Part model, mm, in its own coordinate system. A direction names the side the tool comes from. Round coordinates to 2 decimals unless told otherwise and drop trailing zeros. Loops run counter-clockwise (first coordinate to the right, second up) from the corner with the lowest first, then second, coordinate; pieces in that order, holes last. Notation, with made-up numbers: M -25.75,80.25 L 29.25,80.25 A24 ccw 29.25,111.25 Z; hole C 30,-17.75 d10. An arc over 180 degrees is marked long. Write each question's results on one line, items separated by ' | '.
Autodesk Inventor part; units mm, degrees
ref_plane "YZ Plane" through (0, 0, 0) normal (1, 0, 0) x (0, 1, 0)
ref_plane "XZ Plane" through (0, 0, 0) normal (0, 1, 0) x (-1, 0, 0)
ref_plane "XY Plane" through (0, 0, 0) normal (0, 0, 1) x (1, 0, 0)
sketch "Base" plane through (0, 0, 0) normal (0, 0, 1) x (1, 0, 0)
  line L0 (0, 0) -> (-33.5334, -57.9479)
  line L1 (22.7363, 2.3748) -> (0, 0)
  line L2 (68.7163, -13.2577) -> (22.7363, 2.3748)
  line L3 (-33.5334, -57.9479) -> (-26.9158, -67.5067)
  line L4 (-26.9158, -67.5067) -> (-51.547, -128.5125)
  line L5 (-51.547, -128.5125) -> (-33.4114, -135.8348)
  line L6 (-26.9158, -67.5067) -> (12.6221, -101.6388) construction
  line L7 (12.6221, -101.6388) -> (22.7363, -101.0656)
  line L8 (12.6221, -101.6388) -> (-8.1441, -124.1457)
  line L9 (-33.4114, -135.8348) -> (-8.1441, -124.1457)
  line L10 (22.7363, 2.3748) -> (68.7163, -13.2577)
  line L11 (68.7163, -13.2577) -> (112.7039, -111.8391)
  line L12 (22.7363, 2.3748) -> (22.7363, -101.0656) construction
  line L13 (22.7363, -101.0656) -> (65.9464, -171.4033)
  line L14 (112.7039, -111.8391) -> (105.2475, -122.1197)
  line L15 (22.7363, -101.0656) -> (112.7039, -111.8391) construction
  line L16 (105.2475, -122.1197) -> (103.571, -134.8197)
  line L17 (103.571, -134.8197) -> (108.4402, -146.5492)
  line L18 (65.9464, -171.4033) -> (74.9694, -180.3406)
  line L19 (108.4402, -146.5492) -> (74.9694, -180.3406)
  circle A0 centre (85.3652, -157.1655) radius 25.4
  line L20 (-42.4792, -132.1736) -> (22.7363, -49.3454) construction
  line L21 (-33.0514, -120.1997) -> (-25.1949, -110.2215) construction
  line L22 (-35.546, -118.2356) -> (-27.6895, -108.2573)
  line L23 (-22.7004, -112.1856) -> (-30.5568, -122.1638)
  arc A1 (-35.546, -118.2356) -> (-30.5568, -122.1638) centre (-33.0514, -120.1997) ccw
  arc A2 (-22.7004, -112.1856) -> (-27.6895, -108.2573) centre (-25.1949, -110.2215) ccw
  circle A3 centre (85.3652, -157.1655) radius 4
  line L24 (0, -219.5535) -> (0, 39.3628)
  point P0 (-29.1232, -115.2106)
  point P1 (60.5618, -162.6381)
  dimension "d4" = 50.8
  dimension "d5" = 22.86
  dimension "d6" = 155.26
  dimension "d7" = 126.02
  dimension "d8" = 48.5647
  dimension "d9" = 66.9511
  dimension "d10" = 132.824
  dimension "d11" = 107.95
  dimension "d12" = 115.248
  dimension "d13" = 11.6259
  dimension "d14" = 65.7906
  dimension "d15" = 19.558
  dimension "d16" = 120
  dimension "d17" = 12.7
  dimension "d18" = 12.7
  dimension "d19" = 12.7
  dimension "d20" = 82.55
  dimension "d21" = 12.7
  dimension "d24" = 15.24
  dimension "d25" = 3.175
  dimension "d26" = 12.7
  dimension "d31" = 8
  dimension "d32" = 95.963
  dimension "d33" = 38.215
  dimension "d34" = 22.545
  dimension "d35" = 7.52
  dimension "d36" = 44.727
  dimension "d37" = 31.563
  dimension "d38" = 86.757
  dimension "d39" = 42.697
  dimension "d40" = 49.197
  dimension "d41" = 114.826
  dimension "d47" = 105.4209
  dimension "d48" = 62.051
extrude "Plate1" add sketch "Base" along normal blind 5
fillet "OutsideFilletsFeature" radius 6.35 14 edges at (68.7163, -13.2577, 2.5) (22.7363, 2.3748, 2.5) (0, 0, 2.5) (-33.5334, -57.9479, 2.5) (-26.9158, -67.5067, 2.5) (-51.547, -128.5125, 2.5) (-33.4114, -135.8348, 2.5) (-8.1441, -124.1457, 2.5) (12.6221, -101.6388, 2.5) (22.7363, -101.0656, 2.5) (60.5618, -162.6381, 2.5) (103.571, -134.8197, 2.5) (105.2475, -122.1197, 2.5) (112.7039, -111.8391, 2.5)
sketch "MountHoles" plane through (0, 0, 5) normal (0, 0, 1) x (1, 0, 0)
  line L0 (-1.6199, -2.7989) -> (-30.9807, -53.5288) construction
  arc A0 (3.2163, 0.3359) -> (-1.6199, -2.7989) centre (3.876, -5.9797) ccw construction
  line L1 (21.3511, 2.2301) -> (3.2163, 0.3359) construction
  arc A1 (24.0549, 1.9264) -> (21.3511, 2.2301) centre (22.0108, -4.0856) ccw construction
  arc A2 (69.8461, -15.7897) -> (66.0912, -12.3652) centre (64.0472, -18.3772) ccw construction
  line L2 (24.0548, 1.9265) -> (66.0912, -12.3652) construction
  line L3 (66.0912, -12.3652) -> (24.0548, 1.9265) construction
  line L4 (-20.7142, -54.4632) -> (5.7075, -8.8047) construction
  line L5 (5.7075, -8.8047) -> (21.6681, -7.1377) construction
  line L6 (21.6681, -7.1377) -> (66.0912, -22.2408) construction
  line L7 (-31.5169, -54.4632) -> (-1.6198, -2.7992) construction
  line L8 (3.2166, 0.336) -> (21.3512, 2.2301) construction
  line L9 (24.0548, 1.9265) -> (66.0912, -12.3652) construction
  line L10 (-31.5169, -54.4632) -> (-20.7142, -54.4632) construction
  line L11 (66.0912, -22.2408) -> (66.0912, -12.3652) construction
  circle A3 centre (5.7075, -8.8047) radius 3
  circle A4 centre (21.6681, -7.1377) radius 3
  circle A5 centre (63.2509, -21.2751) radius 3
  point P0 (0, 0)
  dimension "d49" = 9.35
  dimension "d50" = 9.35
  dimension "d51" = 9.35
  dimension "d52" = 6
  dimension "d53" = 6
  dimension "d54" = 6
  dimension "d55" = 3
extrude "MountHolesFeature" cut sketch "MountHoles" against normal blind 5
sketch "Sketch5" plane through (0, 0, 5) normal (0, 0, 1) x (1, 0, 0)
  circle A0 centre (85.3652, -157.1655) radius 4 construction
  circle A1 centre (85.3652, -157.1655) radius 4
  circle A2 centre (85.3652, -157.1655) radius 19.5 construction
  line L0 (85.3652, -157.1655) -> (95.5724, -173.7807) construction
  line L1 (60.034, -161.7789) -> (24.7209, -104.2961) construction
  line L2 (85.3652, -157.1655) -> (101.9804, -146.9584) construction
  circle A3 centre (101.9804, -146.9584) radius 1.25
  circle A4 centre (98.7725, -143.0058) radius 1.25
  circle A5 centre (104.0561, -151.6065) radius 1.25
  circle A6 centre (68.75, -167.3726) radius 1.25
  circle A7 centre (66.6744, -162.7245) radius 1.25
  circle A8 centre (71.958, -171.3251) radius 1.25
  point P0 (0, 0)
  dimension "d67" = 39
  dimension "d68" = 2.5
  dimension "d71" = 30
extrude "Cut5" cut sketch "Sketch5" against normal blind 5 contours A3 | A4 | A5 | A6 | A7 | A8
equation "\"d50\" = d49"
equation "\"d51\" = d49"
equation "\"d56\" = Thickness"
equation "\"d42\" = Thickness"
equation "\"BendRadius\" = Thickness"
equation "\"BendReliefWidth\" = Thickness"
equation "\"BendReliefDepth\" = 0.5 * Thickness"
equation "\"TransitionRadius\" = BendRadius"
equation "\"JacobiRadiusSize\" = BendRadius"
equation "\"GapSize\" = Thickness"
properties part number "Knee"
Item 1: Band-saw the part on B-B on y = -36.5. Give the cut face in (x, z).
Filled sheet:
outline: M -21.12,0 L 79.09,0 L 79.09,5 L -21.12,5 Z
Item 2: Band-saw the part on C-C on x = 0.5. Give the cut face in (y, z), and give its area (3 significant figures).
Filled sheet:
outline: M -114.78,0 L -0.6,0 L -0.6,5 L -114.78,5 Z | area: 571 mm^2
Item 3: Drop flat-ended pins along their axis: P1, Ø2, axis at y = -129, z = 3.5, coming from the +X side; P2, Ø1, axis at x = 59, z = 4, coming from the -Y side. Give the stop position or say it passes through.
Filled sheet:
P1: x = 104.47 | P2: y = -160.91
Item 4: Band-saw the part on A-A on z = 1.95. Count the separate pieces of the cut face and the enclosed holes in it, and give its area (3 significant figures).
Filled sheet:
separate pieces: 1 | enclosed holes: 11 | area: 16,800 mm^2
Item 5: Wall check: L1, parallel to Y at x = 8, z = 0.3; L2, parallel to X at y = -157.5, z = 2.55; L3, parallel to X at y = -21, z = 2.9. Give the ranges that are in metal, low to high.
Filled sheet:
L1: -106.65 to -10.74, -6.87 to 0.84 | L2: 57.41 to 81.38, 89.35 to 110.76 | L3: -12.15 to 60.26, 66.24 to 72.17
Item 6: Which spindle directions (+Z, -Z, +X, -X, +Y, -Y) get a long thin tool onto all of the face, cutting with end or side? Do faces 5 (the flat face through (-38.537, -96.29, 2.465)), 6 (the flat face through (-31.673, -113.316, 2.465)), 7 (the flat face through (12.411, 1.296, 2.465)), 8 (the flat face through (1.923, -113.235, 2.465)). Say none if no direction does.
Filled sheet:
face 5: +Z, -Z, -X | face 6: +Z, -Z | face 7: +Z, -Z, -X, +Y | face 8: +Z, -Z, -Y
Item 7: Two-plate mould, pull along Y, no slides. Class faces 1 (the cylindrical face through (-27.77, -67.65, 2.54)), 2 (the flat face through (-16.36, -28.27, 2.46)), 3 (the cylindrical face through (-49.153, -127.42, 2.535)), 4 (the flat face through (42.13, -132.635, 2.465)): +Y half, -Y half, draft (parallel to the pull), parting line (faces both ways), or undercut.
Filled sheet:
face 1: undercut | face 2: +Y half | face 3: parting line | face 4: -Y half
